```python
from build123d import *

# Parameters (mm, degrees)
F0_W      = 180.34
F0_H      = 165.1
F1_DEPTH  = 76.2
F2_W      = 63.5
F2_H      = 27.94
F3_DEPTH  = 25.4
F5_W      = 63.5
F5_H      = 27.94
F6_DEPTH  = 25.4
F7_R      = 4.7625
F8_DEPTH  = 15.24
F9_R      = 4.7625
F10_DEPTH = 15.24


with BuildPart() as f1:
    # F0 (on Front) → F1 (new body)
    with BuildSketch(Plane.XZ):
        with Locations((90.17, 82.55)):
            Rectangle(F0_W, F0_H)
    extrude(amount=F1_DEPTH)

    # F2 (on face) → F3 (cut)
    with BuildSketch(Plane.XY.offset(165.1)):
        with Locations((31.75, -62.23)):
            Rectangle(F2_W, F2_H)
    extrude(amount=-F3_DEPTH, mode=Mode.SUBTRACT)

    # F5 (on face) → F6 (cut)
    with BuildSketch(Plane.XY.offset(165.1)):
        with Locations((148.59, -62.23)):
            Rectangle(F5_W, F5_H)
    extrude(amount=-F6_DEPTH, mode=Mode.SUBTRACT)

    # F7 (on face) → F8 (join)
    with BuildSketch(Plane.XY.offset(139.7)):
        with Locations((25.4, -62.23)):
            Circle(F7_R)
    extrude(amount=F8_DEPTH)

    # F9 (on face) → F10 (join)
    with BuildSketch(Plane.XY.offset(139.7)):
        with Locations((154.94, -62.23)):
            Circle(F9_R)
    extrude(amount=F10_DEPTH)


solid = f1.part
```
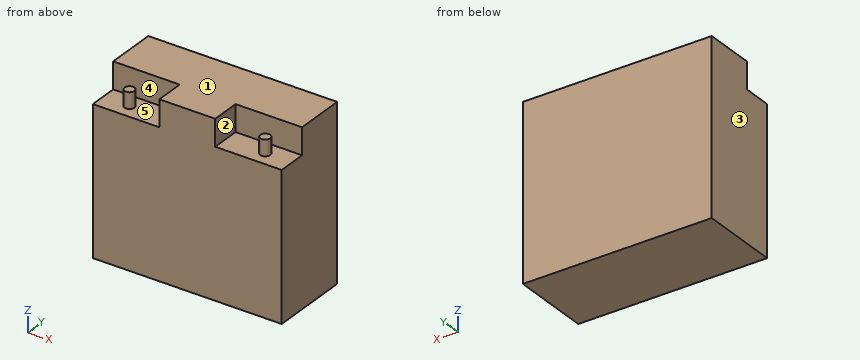
Can you work these out from the model? Positions are in its coordinate system, mm. Face numbers are marked on the shaded views. A direction names the side the tool comes from. Give positions to 0.01 mm unless a question says otherwise; leave off trailing zeros. Loops run counter-clockwise (first coordinate to the right, second up) from the corner with the lowest first, then second, coordinate; pieces in that order, holes last. Notation, with made-up numbers: M 85.5,28 L 135.5,28 A6 cw 135.5,33 Z; hole C 68.5,87 d7. An arc over 180 degrees is marked long. Use CSV: the item, a comma, the result in double quotes. Start each with the question number.
1. Imagine slicing it at A-A, the plane x = 25.4. Write out the boundary of the cut face in (y, z), plus the area to 3 significant figures.
2. On a 3-axis mill with a long thin cutter (end or side, diameter ignored), from which of +Z, -Z, +X, -X, +Y, -Y can I reach the whole of each face in a straight line? I mean the marked faces 1 and 2. Say none if no direction works.
3. Imagine slicing it at B-B, the plane x = 164. Write out the boundary of the cut face in (y, z), plus the area to 3 significant figures.
4. If we mould it in two halves opening along X, with no side actions, what happens to the marked faces 3, 4 and 5? For each: released by +X, released by -X, zero draft, split by the parting line, or undercut.
5. For P1, Ø12, axis at x = 148, y = -55, coming from the +Z side; P2, Ø20.5, axis at x = 33.5, z = 157, coming from the -Y side; P3, Ø7.5, axis at x = 160.5, z = 154.5, coming from the -Y side, each with a flat end and sliding along its axis, tell me the tip position at first contact or that it passes through.
6. If I drill on L1, parallel to Y at x = 57.5, z = 153; L2, parallel to Z at x = 17, y = -63.5, over which ranges is the centre line in solid material (lowest first)?
Response values:
1,outline,"M -76.2,0 L 0,0 L 0,165.1 L -48.26,165.1 L -48.26,139.7 L -57.47,139.7 L -57.47,154.94 L -66.99,154.94 L -66.99,139.7 L -76.2,139.7 Z"
1,area,"12,000 mm^2"
2,face 1,"+Z, +X, -X, +Y, -Y"
2,face 2,"+Z, -Y"
3,outline,"M -76.2,0 L 0,0 L 0,165.1 L -48.26,165.1 L -48.26,139.7 L -76.2,139.7 Z"
3,area,"11,900 mm^2"
4,face 3,"released by -X"
4,face 4,"zero draft"
4,face 5,"undercut"
5,P1,"z = 154.94"
5,P2,"y = -66.99"
5,P3,"y = -66.64"
6,L1,"-48.26 to 0"
6,L2,"0 to 139.7"
